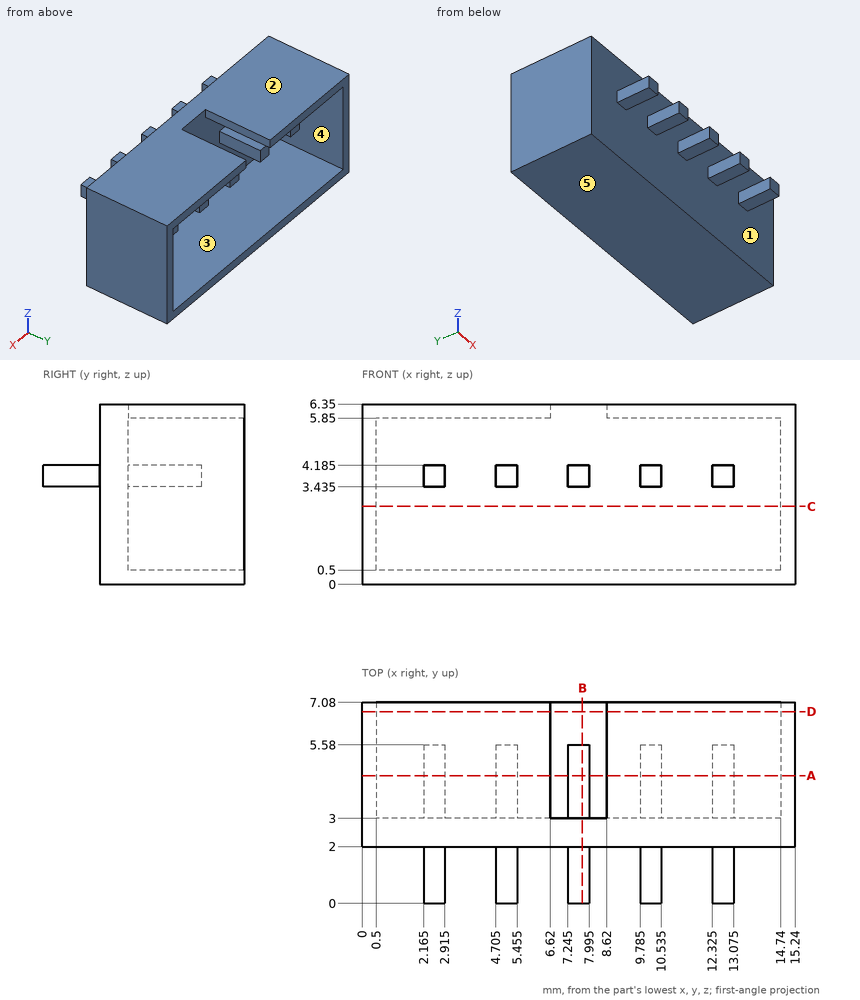
Geometry check sheet. Reference: drawing and pictorial views, mm from the part's lowest x, y, z. A direction names the side the tool comes from. Coordinates: 2 decimals unless noted, no trailing zeros. Order: outer loops, then holes, each group sorted by start corner. A loop starts at its lowest first (then second) coordinate and runs counter-clockwise, first axis right, second up. Notation, with made-up numbers: (76, -24) -> (122, -24) arc R32 cw to (122, 9) -> close; hole circle Ø6 at (-35.5, 37.25). An arc over 180 degrees is marked (long way). Write item = value, one per line. Start each with the question number.
1) Access from +Z, -Z, +X, -X, +Y, -Y to the whole of each face (thin tool, end or side, straight path). Record for the marked faces 4 and 5.
2) Cross-section at B-B (x = 7.75). Enter the section's corners in (y, z) (3 decimals), then the cut area to 3 significant figures.
3) Cross-section at A-A (y = 4.5). State how many separate pieces and enclosed holes the cut face has, then the cut area to 3 significant figures.
4) Material ranges on L1, parallel to Z at x = 5.5, y = 5.25; L2, parallel to X at y = 3.75, z = 2.5; L3, parallel to Y at x = 6.5, z = 4.5, recorded low to high.
5) Cross-section at C-C (z = 2.75). Enter the section's corners in (x, y).
6) Cross-section at D-D (y = 6.75). Enter the section's corners in (x, z), then the cut area to 3 significant figures.
7) Go/stop test with flat-tipped pins: P1, Ø0.6, axis at x = 8, z = 3.5, coming from the +Y side; P2, Ø1.5, axis at x = 8.5, z = 2, coming from the +Y side; P3, Ø0.8, axis at x = 2.5, y = 1, coming from the +Z side (3 decimals). Record where each tip stops, or that it passes through.
8) Mould release check, pull along Z, two halves, no side actions. Record for the marked faces 1, 2 and 3: +Z half, -Z half, draft (parallel to the pull), parting line (faces both ways), or undercut.
Ans:
q1.face_4 = +Y
q1.face_5 = -Z, +X, -X, +Y, -Y
q2.outline = (0, 3.435) -> (2, 3.435) -> (2, 0) -> (7.08, 0) -> (7.08, 0.5) -> (3, 0.5) -> (3, 3.435) -> (5.58, 3.435) -> (5.58, 4.185) -> (3, 4.185) -> (3, 6.35) -> (2, 6.35) -> (2, 4.185) -> (0, 4.185) -> close
q2.area = 11.8 mm²
q3.separate_pieces = 6
q3.enclosed_holes = 0
q3.area = 22.4 mm²
q4.L1 = 0 to 0.5, 5.85 to 6.35
q4.L2 = 0 to 0.5, 14.74 to 15.24
q4.L3 = 2 to 3
q5.outline = (0, 2) -> (15.24, 2) -> (15.24, 7.08) -> (14.74, 7.08) -> (14.74, 3) -> (0.5, 3) -> (0.5, 7.08) -> (0, 7.08) -> close
q6.outline = (0, 0) -> (15.24, 0) -> (15.24, 6.35) -> (8.62, 6.35) -> (8.62, 5.85) -> (14.74, 5.85) -> (14.74, 0.5) -> (0.5, 0.5) -> (0.5, 5.85) -> (6.62, 5.85) -> (6.62, 6.35) -> (0, 6.35) -> close
q6.area = 19.6 mm²
q7.P1 = 5.58
q7.P2 = 3
q7.P3 = 4.185
q8.face_1 = draft
q8.face_2 = +Z half
q8.face_3 = undercut
